Build history of the part. All positions in model axes, mm. A direction names the side the tool comes from. Give positions to 0.01 mm unless a question says otherwise; leave off trailing zeros. Order: outer loops, then holes, each group sorted by start corner. A loop starts at its lowest first (then second) coordinate and runs counter-clockwise, first axis right, second up. Notation, with made-up numbers: (72, -14.75) - (127, -14.75) arc R13 ccw to (127, 2.25) - close; hole circle Ø8 at (8.25, 27.5). An arc over 180 degrees is marked (long way). One line per item, written item: value.
```python
from build123d import *

# Parameters (mm, degrees)
BOSS_EXTRUDE1_DEPTH            = 70
BOSS_EXTRUDE2_DEPTH            = 70
CUT_EXTRUDE1_DEPTH             = 60
SKETCH13_W                     = 9
SKETCH13_H                     = 60
CUT_EXTRUDE3_DEPTH             = 5
SKETCH12_W                     = 25
SKETCH12_H                     = 23
CUT_EXTRUDE2_DEPTH             = 5
BOSS_EXTRUDE3_DEPTH            = 3.84
CBORE_FOR_M3_SHCS1_D           = 3.4
CBORE_FOR_M3_SHCS1_DEPTH       = 8.05
CBORE_FOR_M3_SHCS1_CBORE_D     = 6.5
CBORE_FOR_M3_SHCS1_CBORE_DEPTH = 4
CBORE_FOR_M3_SHCS1_TIP         = 1.021463052
M3X0_5_TAPPED_HOLE1_D          = 2.5
M3X0_5_TAPPED_HOLE1_DEPTH      = 14
M3X0_5_TAPPED_HOLE1_TIP        = 0.751075774
FILLET1_R                      = 10
FILLET4_R                      = 5
FILLET5_R                      = 3
TOLERANCE_BY                   = 0.05
TOLERANCE_2_BY                 = 0.05
TOLERANCE_3_BY                 = 0.05
TOLERANCE_4_BY                 = 0.05
TOLERANCE_5_BY                 = 0.05
TOLERANCE_6_BY                 = 0.05
TOLERANCE_7_BY                 = 0.05
TOLERANCE_8_BY                 = 0.05


with BuildPart() as part:
    # Sketch3 → Boss-Extrude1 (new body)
    with BuildSketch(Plane.XY):
        with BuildLine():
            Line((85.25, 15), (85.25, 40))
            Line((85.25, 40), (90.25, 40))
            Line((90.25, 40), (90.25, 15))
            ThreePointArc((90.25, 15), (84.392135624, 0.857864376), (70.25, -5))
            Line((70.25, -5), (-12, -5))
            Line((-12, -5), (-12, 60.2))
            Line((-12, 60.2), (0, 60.2))
            Line((0, 60.2), (0, 0))
            Line((0, 0), (70.25, 0))
            ThreePointArc((70.25, 0), (80.856601718, 4.393398282), (85.25, 15))
        make_face()
    extrude(amount=BOSS_EXTRUDE1_DEPTH)

    # Sketch5 → Boss-Extrude2 (add)
    with BuildSketch(Plane.XY.offset(70)):
        with BuildLine():
            Line((82.2, 15), (82.2, 40))
            Line((82.2, 40), (90.25, 40))
            Line((90.25, 40), (90.25, 15))
            ThreePointArc((90.25, 15), (84.392135624, 0.857864376), (70.25, -5))
            Line((70.25, -5), (25.1, -5))
            Line((25.1, -5), (25.1, 40))
            Line((25.1, 40), (33.15, 40))
            Line((33.15, 40), (33.15, 3.05))
            Line((33.15, 3.05), (70.25, 3.05))
            ThreePointArc((70.25, 3.05), (78.699926035, 6.550073965), (82.2, 15))
        make_face()
    extrude(amount=BOSS_EXTRUDE2_DEPTH)

    # Sketch6 → Cut-Extrude1 (cut)
    with BuildSketch(Plane.XY.offset(70)):
        Polygon((-3, 24.26), (0, 26.24), (0, 60.2), (-3, 60.2), align=None)
    extrude(amount=-CUT_EXTRUDE1_DEPTH, mode=Mode.SUBTRACT)

    # Sketch13 → Cut-Extrude3 (cut)
    with BuildSketch(Plane(origin=(0, 60.2, 0), x_dir=(1, 0, 0), z_dir=(0, 1, 0))):
        with Locations((-7.5, -40)):
            Rectangle(SKETCH13_W, SKETCH13_H)
    extrude(amount=-CUT_EXTRUDE3_DEPTH, mode=Mode.SUBTRACT)

    # Sketch12 → Cut-Extrude2 (cut)
    with BuildSketch(Plane(origin=(90.25, 0, 0), x_dir=(0, 0, -1), z_dir=(1, 0, 0))):
        with Locations((-50, 28.5)):
            Rectangle(SKETCH12_W, SKETCH12_H)
    extrude(amount=-CUT_EXTRUDE2_DEPTH, mode=Mode.SUBTRACT)

    # Sketch7 → Boss-Extrude3 (add)
    with BuildSketch(Plane.XY):
        with BuildLine():
            Line((-12, 60.2), (-12, -5))
            Line((-12, -5), (70.25, -5))
            ThreePointArc((70.25, -5), (84.392135624, 0.857864376), (90.25, 15))
            Line((90.25, 15), (90.25, 60.2))
            Line((90.25, 60.2), (-12, 60.2))
        make_face()
        with BuildLine():
            Line((70, 51.37), (40, 51.37))
            ThreePointArc((40, 51.37), (32.928932188, 48.441067812), (30, 41.37))
            Line((30, 41.37), (30, 11.37))
            ThreePointArc((30, 11.37), (32.928932188, 4.298932188), (40, 1.37))
            Line((40, 1.37), (70, 1.37))
            ThreePointArc((70, 1.37), (77.071067812, 4.298932188), (80, 11.37))
            Line((80, 11.37), (80, 41.37))
            ThreePointArc((80, 41.37), (77.071067812, 48.441067812), (70, 51.37))
        make_face(mode=Mode.SUBTRACT)
    extrude(amount=-BOSS_EXTRUDE3_DEPTH)

    # CBORE for M3 SHCS1
    with Locations(Plane(origin=(0, 3.05, 0), x_dir=(1, 0, 0), z_dir=(0, 1, 0))):
        with Locations((40.175, -82.5), (55.175, -82.5)):
            CounterBoreHole(CBORE_FOR_M3_SHCS1_D / 2, CBORE_FOR_M3_SHCS1_CBORE_D / 2, CBORE_FOR_M3_SHCS1_CBORE_DEPTH, depth=CBORE_FOR_M3_SHCS1_DEPTH)
            with Locations((0, 0, -(CBORE_FOR_M3_SHCS1_DEPTH + CBORE_FOR_M3_SHCS1_TIP / 2))):  # 118° drill point
                Cone(0, CBORE_FOR_M3_SHCS1_D / 2, CBORE_FOR_M3_SHCS1_TIP, mode=Mode.SUBTRACT)

    # M3x0.5 Tapped Hole1
    with Locations(Plane(origin=(0, 55.2, 0), x_dir=(1, 0, 0), z_dir=(0, 1, 0))):
        with Locations((-7.5, -25), (-7.5, -55)):
            Hole(M3X0_5_TAPPED_HOLE1_D / 2, depth=M3X0_5_TAPPED_HOLE1_DEPTH)
            with Locations((0, 0, -(M3X0_5_TAPPED_HOLE1_DEPTH + M3X0_5_TAPPED_HOLE1_TIP / 2))):  # 118° drill point
                Cone(0, M3X0_5_TAPPED_HOLE1_D / 2, M3X0_5_TAPPED_HOLE1_TIP, mode=Mode.SUBTRACT)

    # Fillet1
    fillet1_edges = [part.edges().sort_by_distance(p)[0] for p in [
        (25.1, -2.5, 70),
    ]]
    fillet(fillet1_edges, radius=FILLET1_R)

    # Fillet4
    fillet4_edges = [part.edges().sort_by_distance(p)[0] for p in [
        (87.75, 17, 37.5),
        (87.75, 17, 62.5),
    ]]
    fillet(fillet4_edges, radius=FILLET4_R)

    # Fillet5
    fillet5_edges = [part.edges().sort_by_distance(p)[0] for p in [
        (87.75, 40, 0),
        (90.25, 60.2, -1.92),
    ]]
    fillet(fillet5_edges, radius=FILLET5_R)

    # Tolerance: a curved face moved inward by 0.05
    add(Solid.thicken(part.faces().sort_by_distance((32.928932188, 4.298932188, -1.92))[0], -TOLERANCE_BY), mode=Mode.SUBTRACT)

    # Tolerance 2: a face moved inward by 0.05
    extrude(part.faces().sort_by_distance((30, 26.37, -1.92))[0], amount=TOLERANCE_2_BY, dir=(-1, 0, 0), mode=Mode.SUBTRACT)

    # Tolerance 3: a curved face moved inward by 0.05
    add(Solid.thicken(part.faces().sort_by_distance((32.928932188, 48.441067812, -1.92))[0], -TOLERANCE_3_BY), mode=Mode.SUBTRACT)

    # Tolerance 4: a face moved inward by 0.05
    extrude(part.faces().sort_by_distance((55, 51.37, -1.92))[0], amount=TOLERANCE_4_BY, dir=(0, 1, 0), mode=Mode.SUBTRACT)

    # Tolerance 5: a curved face moved inward by 0.05
    add(Solid.thicken(part.faces().sort_by_distance((77.071067812, 48.441067812, -1.92))[0], -TOLERANCE_5_BY), mode=Mode.SUBTRACT)

    # Tolerance 6: a face moved inward by 0.05
    extrude(part.faces().sort_by_distance((80, 26.37, -1.92))[0], amount=TOLERANCE_6_BY, dir=(1, 0, 0), mode=Mode.SUBTRACT)

    # Tolerance 7: a curved face moved inward by 0.05
    add(Solid.thicken(part.faces().sort_by_distance((77.071067812, 4.298932188, -1.92))[0], -TOLERANCE_7_BY), mode=Mode.SUBTRACT)

    # Tolerance 8: a face moved inward by 0.05
    extrude(part.faces().sort_by_distance((55, 1.37, -1.92))[0], amount=TOLERANCE_8_BY, dir=(0, -1, 0), mode=Mode.SUBTRACT)


solid = part.part
```
(1) Slice it at C-C, the plane x = 61. Give the cut face in (y, z), and give its area (3 significant figures).
Completed:
outline: (-5, -3.84) - (1.32, -3.84) - (1.32, 0) - (0, 0) - (0, 70) - (3.05, 70) - (3.05, 140) - (-5, 140) - close; (51.42, -3.84) - (60.2, -3.84) - (60.2, 0) - (51.42, 0) - close
area: 971 mm²
(2) Pull direction Z, two halves, no side cores. Call faces 4 (the face through (86, 40, 101)), 5 (the face through (57, -0.95, 84)), 6 (the face through (22.09, -2.46, 72.85)): +Z half, -Z half, draft (parallel to the pull), parting line (faces both ways), or undercut.
Completed:
face 4: draft
face 5: undercut
face 6: +Z half
(3) Drill centre lines: line 1 (X direction, y = 19, z = 36); line 2 (X direction, y = 31, z = 117); line 3 (X direction, y = 1, z = 82). Where is each one in solid material? Low to high.
Completed:
line 1: -12 to 0, 85.25 to 90.25
line 2: 25.1 to 33.15, 82.2 to 90.25
line 3: 25.1 to 36.96, 43.39 to 51.96, 58.39 to 84.53
(4) Slice it at D-D, the plane y = 36. Give the cut face in (x, z).
Completed:
outline: (-12, -3.84) - (29.95, -3.84) - (29.95, 0) - (0, 0) - (0, 10) - (-3, 10) - (-3, 70) - (-12, 70) - close; (25.1, 70) - (33.15, 70) - (33.15, 140) - (25.1, 140) - close; (80.05, -3.84) - (90.25, -3.84) - (90.25, 37.5) - (85.25, 37.5) - (85.25, 0) - (80.05, 0) - close; (82.2, 70) - (85.25, 70) - (85.25, 62.5) - (90.25, 62.5) - (90.25, 140) - (82.2, 140) - close
(5) Pin check, flat tips, straight feed: P1, Ø12, axis at x = 58, y = 9, coming from the -Z side; P2, Ø2.5, axis at x = 87, z = 27, coming from the +Y side; P3, Ø3, axis at x = 73, z = 33.5, coming from the -Y side. Stop position of each tip, or through.
Completed:
P1: z = 70
P2: y = 40
P3: y = -4.96
(6) Slice it at B-B, the plane z = 82.5. Give the cut face in (x, y) (3 decimals).
Completed:
outline: (25.1, -5) - (38.475, -5) - (38.475, -0.95) - (36.925, -0.95) - (36.925, 3.05) - (33.15, 3.05) - (33.15, 40) - (25.1, 40) - close; (41.875, -5) - (53.475, -5) - (53.475, -0.95) - (51.925, -0.95) - (51.925, 3.05) - (43.425, 3.05) - (43.425, -0.95) - (41.875, -0.95) - close; (56.875, -5) - (70.25, -5) arc R20 ccw to (90.25, 15) - (90.25, 40) - (82.2, 40) - (82.2, 15) arc R11.95 cw to (70.25, 3.05) - (58.425, 3.05) - (58.425, -0.95) - (56.875, -0.95) - close
(7) 3-axis set-ups, long thin cutter, end or side, ignore diameter. For faces 1 (the face through (88, 31, 37.5)), 2 (the face through (-8, 55.2, 40)), 3 (the face through (32.97, 48.55, -1.89)): which of +Z, -Z, +X, -X, +Y, -Y reach the whole face in a straight line?
Completed:
face 1: +X, +Y
face 2: +Z, +X, -X, +Y
face 3: +Z, -Z
(8) Slice it at A-A, the plane y = 49. Give the cut face in (x, z), and give its area (3 significant figures).
Completed:
outline: (-12, -3.84) - (33.46, -3.84) - (33.46, 0) - (0, 0) - (0, 10) - (-3, 10) - (-3, 70) - (-12, 70) - close; (76.54, -3.84) - (90.25, -3.84) - (90.25, 0) - (76.54, 0) - close; hole circle Ø2.5 at (-7.5, 25); hole circle Ø2.5 at (-7.5, 55)
area: 877 mm²
